The listing builds one solid part. Answer for the finished solid, in the listing's coordinates (mm). Round coordinates to 2 decimals unless told otherwise and drop trailing zeros. Order: outer loops, then holes, each group sorted by start corner. A loop starts at its lowest first (then second) coordinate and runs counter-clockwise, first axis right, second up. Notation, with made-up numbers: M -12.75,-8 L -0.75,-8 A20 ccw -0.75,23 Z; hole C 49,1 d4. An arc over 180 degrees is marked long. Write item = value, one per line. Start each with the question number.
(1) A cutting plane is placed at B-B, the plane x = 185. Determine the outline of the cut face in (y, z).
(2) A cutting plane is placed at A-A, the plane y = 2. Count the separate pieces of the cut face and the enclosed holes in it, and give its area (3 significant figures).
(3) Straight lines are drawn through the part: probe 1 along Z at (x, y) = (142, 7.25); probe 2 along X at (y, z) = (4, -6); probe 3 along X at (y, z) = (5, 5.5). For each, find the intervals that lie inside material, in ascending order. Write a range as from..to.
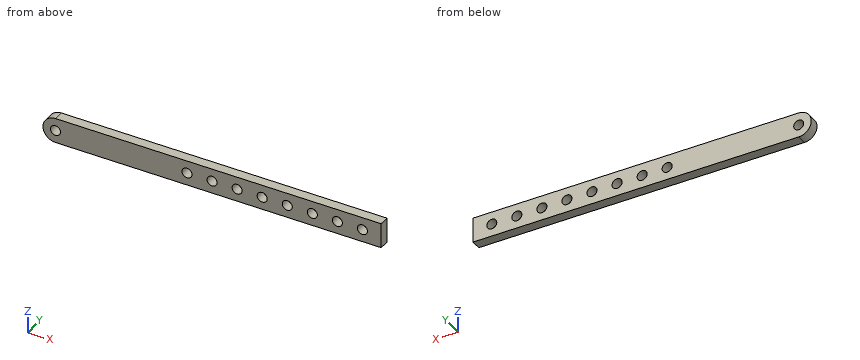
from build123d import *

# Parameters (mm, degrees)
BOSS_EXTRUDE1_DEPTH = 8
SKETCH2_R           = 4
CUT_EXTRUDE1_DEPTH  = 8
SKETCH3_R           = 4
CUT_EXTRUDE2_DEPTH  = 10
LPATTERN1_COUNT     = 8
LPATTERN1_PITCH     = 20


with BuildPart() as part:
    # Sketch1 → Boss-Extrude1 (new body)
    with BuildSketch(Plane(origin=(0, 0, 0), x_dir=(1, 0, 0), z_dir=(0, 1, 0))):
        with BuildLine():
            Line((0, 10), (260, 10))
            Line((260, 10), (260, -10))
            Line((260, -10), (0, -10))
            ThreePointArc((0, -10), (-10, 0), (0, 10))
        make_face()
    extrude(amount=BOSS_EXTRUDE1_DEPTH)

    # Sketch2 → Cut-Extrude1 (cut)
    with BuildSketch(Plane(origin=(0, 8, 0), x_dir=(1, 0, 0), z_dir=(0, 1, 0))):
        with Locations(Location((0, 0, 0), (0, 0, 270))):
            Circle(SKETCH2_R)
    extrude(amount=-CUT_EXTRUDE1_DEPTH, mode=Mode.SUBTRACT)

    # Sketch3 → Cut-Extrude2 (cut)
    with BuildSketch(Plane(origin=(0, 8, 0), x_dir=(1, 0, 0), z_dir=(0, 1, 0))):
        with Locations(Location((245, 0, 0), (0, 0, 270))):
            Circle(SKETCH3_R)
    cut_extrude2 = extrude(amount=-CUT_EXTRUDE2_DEPTH, mode=Mode.SUBTRACT)

    # LPattern1: Cut-Extrude2 ×8
    with Locations(*[(-i * LPATTERN1_PITCH, 0, 0) for i in range(1, LPATTERN1_COUNT)]):
        add(cut_extrude2, mode=Mode.SUBTRACT)


solid = part.part
Reported:
q1.outline = M 0,-10 L 8,-10 L 8,-4 L 0,-4 Z; M 0,4 L 8,4 L 8,10 L 0,10 Z
q2.separate_pieces = 1
q2.enclosed_holes = 9
q2.area = 4,900 mm²
q3.probe_1 = -10..-2.65, 2.65..10
q3.probe_2 = -8..260
q3.probe_3 = -8.35..260
